from build123d import *

# Parameters (mm, degrees)
SKETCH1_R           = 16
BOSS_EXTRUDE1_DEPTH = 6.5
BOSS_EXTRUDE2_DEPTH = 3
SKETCH3_R           = 1.5
BOSS_EXTRUDE3_DEPTH = 10
SKETCH4_R           = 14
CUT_EXTRUDE1_DEPTH  = 7.5
SKETCH5_R           = 1.5
CUT_EXTRUDE2_DEPTH  = 54.986109325


with BuildPart() as part:
    # Sketch1 → Boss-Extrude1 (new body)
    with BuildSketch(Plane(origin=(0, 0, 0), x_dir=(1, 0, 0), z_dir=(0, 1, 0))):
        with Locations(Location((0, 0, 0), (0, 0, 90))):
            Circle(SKETCH1_R)
    extrude(amount=BOSS_EXTRUDE1_DEPTH)

    # Sketch2 → Boss-Extrude2 (add)
    with BuildSketch(Plane(origin=(0, 6.5, 0), x_dir=(1, 0, 0), z_dir=(0, 1, 0))):
        with BuildLine():
            Line((-16, -32.5), (-16, 32.5))
            ThreePointArc((-16, 32.5), (0, 48.5), (16, 32.5))
            Line((16, 32.5), (16, -32.5))
            ThreePointArc((16, -32.5), (0, -48.5), (-16, -32.5))
        make_face()
    extrude(amount=BOSS_EXTRUDE2_DEPTH)

    # Sketch3 → Boss-Extrude3 (add)
    with BuildSketch(Plane(origin=(0, 9.5, 0), x_dir=(1, 0, 0), z_dir=(0, 1, 0))):
        with Locations(Location((0, 32.5, 0), (0, 0, 270))):
            Circle(SKETCH3_R)
        with Locations(Location((0, -32.5, 0), (0, 0, 270))):
            Circle(SKETCH3_R)
    extrude(amount=BOSS_EXTRUDE3_DEPTH)

    # Sketch4 → Cut-Extrude1 (cut)
    with BuildSketch(Plane(origin=(0, 9.5, 0), x_dir=(1, 0, 0), z_dir=(0, 1, 0))):
        with Locations(Location((0, 0, 0), (0, 0, 270))):
            Circle(SKETCH4_R)
    extrude(amount=-CUT_EXTRUDE1_DEPTH, mode=Mode.SUBTRACT)

    # Sketch5 → Cut-Extrude2 (cut, through all)
    with BuildSketch(Plane(origin=(0, 2, 0), x_dir=(1, 0, 0), z_dir=(0, 1, 0))):
        with Locations(Location((8, 0, 0), (0, 0, 270))):
            Circle(SKETCH5_R)
        with Locations(Location((0, -8, 0), (0, 0, 270))):
            Circle(SKETCH5_R)
        with Locations(Location((-8, 0, 0), (0, 0, 270))):
            Circle(SKETCH5_R)
        with Locations(Location((0, 8, 0), (0, 0, 270))):
            Circle(SKETCH5_R)
    extrude(amount=-CUT_EXTRUDE2_DEPTH, mode=Mode.SUBTRACT)


solid = part.part
Build history of the part. All positions in model axes, mm. A direction names the side the tool comes from. Round coordinates to 2 decimals unless told otherwise and drop trailing zeros. Write each loop counter-clockwise with the first axis right and the second up, starting at its lowest first coordinate (ties: lowest second). Pieces come first, ordered by that corner, then holes. Notation, with made-up numbers: (-22.75, 14) - (-7.75, 14) arc R12 cw to (-7.75, 27) - close; hole circle Ø7 at (-15.5, 5.25). An arc over 180 degrees is marked (long way). One line per question, with ' | ' between items.
1. Drill centre lines: line 1 along X through (y, z) = (1.05, 0); line 2 along Y through (x, z) = (10, 39); line 3 along Y through (x, z) = (-7, 6.5). Where is each one in solid material? Low to high. Write a range as from..to.
Results are:
line 1: -16..-9.5, -6.5..6.5, 9.5..16 | line 2: 6.5..9.5 | line 3: 0..2
2. Band-saw the part on B-B, the plane x = -8. Write the cut outline in (y, z).
Results are:
outline: (0, -13.86) - (6.5, -13.86) - (6.5, -46.36) - (9.5, -46.36) - (9.5, -11.49) - (2, -11.49) - (2, -1.5) - (0, -1.5) - close; (0, 1.5) - (2, 1.5) - (2, 11.49) - (9.5, 11.49) - (9.5, 46.36) - (6.5, 46.36) - (6.5, 13.86) - (0, 13.86) - close
3. Drop flat-ended pins along their axis: pin 1 Ø1 at (x, y) = (-4.5, 2.5) entering from +Z; pin 2 Ø1.5 at (x, z) = (-7, -22.5) entering from +Y; pin 3 Ø5 at (x, z) = (3, -28.5) entering from -Y. Give the stop position or say it passes through.
Results are:
pin 1: z = 15.49 | pin 2: y = 9.5 | pin 3: y = 6.5
4. Band-saw the part on A-A, the plane x = 0. Write the cut outline in (y, z).
Results are:
outline: (0, -16) - (6.5, -16) - (6.5, -48.5) - (9.5, -48.5) - (9.5, -34) - (19.5, -34) - (19.5, -31) - (9.5, -31) - (9.5, -14) - (2, -14) - (2, -9.5) - (0, -9.5) - close; (0, -6.5) - (2, -6.5) - (2, 6.5) - (0, 6.5) - close; (0, 9.5) - (2, 9.5) - (2, 14) - (9.5, 14) - (9.5, 31) - (19.5, 31) - (19.5, 34) - (9.5, 34) - (9.5, 48.5) - (6.5, 48.5) - (6.5, 16) - (0, 16) - close
5. Band-saw the part on D-D, the plane z = 8. Write the cut outline in (x, y), and give its area (3 significant figures).
Results are:
outline: (-16, 6.5) - (-13.86, 6.5) - (-13.86, 0) - (-1.5, 0) - (-1.5, 2) - (-11.49, 2) - (-11.49, 9.5) - (-16, 9.5) - close; (1.5, 0) - (13.86, 0) - (13.86, 6.5) - (16, 6.5) - (16, 9.5) - (11.49, 9.5) - (11.49, 2) - (1.5, 2) - close | area: 97.8 mm^2
6. Band-saw the part on C-C, the plane y = 15. Write the cut outline in (x, z), and give its area (3 significant figures).
Results are:
outline: circle Ø3 at (0, -32.5); circle Ø3 at (0, 32.5) | area: 14.1 mm^2
7. Mould opens along X. For faces 1 (the face through (-16, 8, 0)), 2 (the face through (0, 19.5, -33)), 3 (the face through (-9.464, 1.014, -0.325)) say: released by +X, released by -X, zero draft, split by the parting line, or undercut.
Results are:
face 1: released by -X | face 2: zero draft | face 3: undercut
8. Tool access for faces 4 (the face through (15.62, 3.2, 3.47)), 5 (the face through (-0.9, 14.4, -33.7)), 6 (the face through (0.352, 7.979, 48.496)): list every direction of +Z, -Z, +X, -X, +Y, -Y with a clear straight run to the whole face (end or side of a thin tool).
Results are:
face 4: -Y | face 5: +Y | face 6: +Z, +Y, -Y
